```python
from build123d import *

# Parameters (mm, degrees)
F1_DEPTH = 23
F2_DEPTH = 22
F0_W     = 12
F0_H     = 10
F0_R     = 3.5
F3_DEPTH = 16
F4_DEPTH = 18
F5_R     = 0.5
F6_DEPTH = 5


with BuildPart() as f1:
    # F0 (on Top) → F1 (new body)
    with BuildSketch(Plane.XY):
        with BuildLine():
            Line((60, 45), (30, 45))
            Line((30, 45), (30, 41.5))
            Line((30, 41.5), (46, 41.5))
            Line((46, 41.5), (46, 31.5))
            Line((46, 31.5), (46, 22.5))
            Line((46, 22.5), (54.5, 22.5))
            ThreePointArc((54.5, 22.5), (56.1109127035, 26.3890872965), (60, 28))
            Line((60, 28), (60, 31.5))
            Line((60, 31.5), (48, 31.5))
            Line((48, 31.5), (48, 41.5))
            Line((48, 41.5), (60, 41.5))
            Line((60, 41.5), (60, 45))
        make_face()
        with BuildLine():
            Line((54.5, 22.5), (46, 22.5))
            Line((46, 22.5), (46, 13.5))
            Line((46, 13.5), (46, 3.5))
            Line((46, 3.5), (30, 3.5))
            Line((30, 3.5), (30, 0))
            Line((30, 0), (60, 0))
            Line((60, 0), (60, 3.5))
            Line((60, 3.5), (48, 3.5))
            Line((48, 3.5), (48, 13.5))
            Line((48, 13.5), (60, 13.5))
            Line((60, 13.5), (60, 17))
            ThreePointArc((60, 17), (56.1109127035, 18.6109127035), (54.5, 22.5))
        make_face()
        with BuildLine():
            Line((14, 13.5), (14, 22.5))
            Line((14, 22.5), (5.5, 22.5))
            ThreePointArc((5.5, 22.5), (3.8890872965, 18.6109127035), (0, 17))
            Line((0, 17), (0, 13.5))
            Line((0, 13.5), (12, 13.5))
            Line((12, 13.5), (12, 3.5))
            Line((12, 3.5), (0, 3.5))
            Line((0, 3.5), (0, 0))
            Line((0, 0), (30, 0))
            Line((30, 0), (30, 3.5))
            Line((30, 3.5), (14, 3.5))
            Line((14, 3.5), (14, 13.5))
        make_face()
        with BuildLine():
            Line((30, 45), (0, 45))
            Line((0, 45), (0, 41.5))
            Line((0, 41.5), (6, 41.5))
            Line((6, 41.5), (12, 41.5))
            Line((12, 41.5), (12, 31.5))
            Line((12, 31.5), (6, 31.5))
            Line((6, 31.5), (0, 31.5))
            Line((0, 31.5), (0, 28))
            ThreePointArc((0, 28), (3.8890872965, 26.3890872965), (5.5, 22.5))
            Line((5.5, 22.5), (14, 22.5))
            Line((14, 22.5), (14, 31.5))
            Line((14, 31.5), (14, 41.5))
            Line((14, 41.5), (30, 41.5))
            Line((30, 41.5), (30, 45))
        make_face()
    extrude(amount=F1_DEPTH)

    # F0 (on Top) → F2 (join)
    with BuildSketch(Plane.XY):
        Polygon((30, 22.5), (30, 41.5), (14, 41.5), (14, 31.5), (14, 22.5), align=None)
        Polygon((46, 41.5), (30, 41.5), (30, 22.5), (46, 22.5), (46, 31.5), align=None)
        Polygon((46, 22.5), (30, 22.5), (30, 3.5), (46, 3.5), (46, 13.5), align=None)
        Polygon((30, 3.5), (30, 22.5), (14, 22.5), (14, 13.5), (14, 3.5), align=None)
    extrude(amount=F2_DEPTH)

    # F0 (on Top) → F3 (join)
    with BuildSketch(Plane.XY):
        with BuildLine():
            Line((6, 41.5), (0, 41.5))
            Line((0, 41.5), (0, 31.5))
            Line((0, 31.5), (6, 31.5))
            Line((6, 31.5), (6, 33))
            ThreePointArc((6, 33), (2.5, 36.5), (6, 40))
            Line((6, 40), (6, 41.5))
        make_face()
        with BuildLine():
            Line((12, 41.5), (6, 41.5))
            Line((6, 41.5), (6, 40))
            ThreePointArc((6, 40), (8.4748737342, 38.9748737342), (9.5, 36.5))
            ThreePointArc((9.5, 36.5), (8.4748737342, 34.0251262658), (6, 33))
            Line((6, 33), (6, 31.5))
            Line((6, 31.5), (12, 31.5))
            Line((12, 31.5), (12, 41.5))
        make_face()
        with Locations((6, 8.5)):
            Rectangle(F0_W, F0_H)
        with Locations((6, 8.5)):
            Circle(F0_R, mode=Mode.SUBTRACT)
        with Locations((54, 36.5)):
            Rectangle(F0_W, F0_H)
        with Locations((54, 36.5)):
            Circle(F0_R, mode=Mode.SUBTRACT)
        with Locations((54, 8.5)):
            Rectangle(F0_W, F0_H)
        with Locations((54, 8.5)):
            Circle(F0_R, mode=Mode.SUBTRACT)
    extrude(amount=F3_DEPTH)

    # F0 (on Top) → F4 (join)
    with BuildSketch(Plane.XY):
        with BuildLine():
            ThreePointArc((9.5, 36.5), (8.4748737342, 38.9748737342), (6, 40))
            Line((6, 40), (6, 33))
            ThreePointArc((6, 33), (8.4748737342, 34.0251262658), (9.5, 36.5))
        make_face()
        with BuildLine():
            Line((6, 33), (6, 40))
            ThreePointArc((6, 40), (2.5, 36.5), (6, 33))
        make_face()
        with Locations((6, 8.5)):
            Circle(F0_R)
        with Locations((54, 36.5)):
            Circle(F0_R)
        with Locations((54, 8.5)):
            Circle(F0_R)
    extrude(amount=F4_DEPTH)

    # F5
    f5_edges = [f1.edges().sort_by_distance(p)[0] for p in [
        (2.5, 36.5, 18),
        (2.5, 8.5, 18),
        (50.5, 36.5, 18),
        (50.5, 8.5, 18),
    ]]
    fillet(f5_edges, radius=F5_R)

    # F0 (on Top) → F6 (join)
    with BuildSketch(Plane.XY):
        with BuildLine():
            ThreePointArc((5.5, 22.5), (3.8890872965, 26.3890872965), (0, 28))
            Line((0, 28), (0, 22.5))
            Line((0, 22.5), (5.5, 22.5))
        make_face()
        with BuildLine():
            Line((5.5, 22.5), (0, 22.5))
            Line((0, 22.5), (0, 17))
            ThreePointArc((0, 17), (3.8890872965, 18.6109127035), (5.5, 22.5))
        make_face()
        with BuildLine():
            Line((60, 22.5), (60, 28))
            ThreePointArc((60, 28), (56.1109127035, 26.3890872965), (54.5, 22.5))
            Line((54.5, 22.5), (60, 22.5))
        make_face()
        with BuildLine():
            Line((60, 22.5), (54.5, 22.5))
            ThreePointArc((54.5, 22.5), (56.1109127035, 18.6109127035), (60, 17))
            Line((60, 17), (60, 22.5))
        make_face()
    extrude(amount=F6_DEPTH)


solid = f1.part
```
Read the model definition and answer for the solid it produces. Units are mm, in the model's axes. A direction names the side the tool comes from. Give positions to 0.01 mm unless a question says otherwise; leave off trailing zeros. Order: outer loops, then holes, each group sorted by start corner. A loop starts at its lowest first (then second) coordinate and runs counter-clockwise, first axis right, second up. Notation, with made-up numbers: (33, 10.25) -> (72, 10.25) arc R26 cw to (72, 39.25) -> close; hole circle Ø2 at (69, 75.25). An arc over 180 degrees is marked (long way). Write item = value, one per line.
1. A cutting plane is placed at B-B, the plane z = 18.75. Write down the section's boundary in (x, y).
Numbers:
outline = (0, 0) -> (60, 0) -> (60, 3.5) -> (48, 3.5) -> (48, 13.5) -> (60, 13.5) -> (60, 17) arc R5.5 cw to (60, 28) -> (60, 31.5) -> (48, 31.5) -> (48, 41.5) -> (60, 41.5) -> (60, 45) -> (0, 45) -> (0, 41.5) -> (12, 41.5) -> (12, 31.5) -> (0, 31.5) -> (0, 28) arc R5.5 cw to (0, 17) -> (0, 13.5) -> (12, 13.5) -> (12, 3.5) -> (0, 3.5) -> close
2. A cutting plane is placed at D-D, the plane y = 18. Write down the section's boundary in (x, z).
Numbers:
outline = (0, 0) -> (60, 0) -> (60, 5) -> (56.84, 5) -> (56.84, 23) -> (46, 23) -> (46, 22) -> (14, 22) -> (14, 23) -> (3.16, 23) -> (3.16, 5) -> (0, 5) -> close
3. Given pin 1 (2 mm diameter, centred on y = 37, z = 18.5, fed in from -X); pin 2 (3 mm diameter, centred on x = 55.5, y = 8.5, fed in from +Z); pin 3 (0.5 mm diameter, centred on y = 18.5, z = 22.5, fed in from +X), each flat-ended and moving along its own axis, determine where each tip first touches the part or whether it passes through.
Numbers:
pin_1 = 2.51
pin_2 = 18
pin_3 = 56.51
4. For faces 5 (the face through (3, 39, 16)), 6 (the face through (12, 21, 23)), 7 (the face through (2, 23, 5)), 8 (the face through (54, 9, 18)), determine the directions among +Z, -Z, +X, -X, +Y, -Y from which every point of the face is accessible in a straight line to the end or side of a thin tool.
Numbers:
face_5 = +Z
face_6 = +Z, +X, -X, +Y, -Y
face_7 = +Z, -X
face_8 = +Z, +X
5. A cutting plane is placed at C-C, the plane y = 8.5. Write down the section's boundary in (x, z), and give its area (3 significant figures).
Numbers:
outline = (0, 0) -> (60, 0) -> (60, 16) -> (57.5, 16) -> (57.5, 17.5) arc R0.5 ccw to (57, 18) -> (51, 18) arc R0.5 ccw to (50.5, 17.5) -> (50.5, 16) -> (48, 16) -> (48, 23) -> (46, 23) -> (46, 22) -> (14, 22) -> (14, 23) -> (12, 23) -> (12, 16) -> (9.5, 16) -> (9.5, 17.5) arc R0.5 ccw to (9, 18) -> (3, 18) arc R0.5 ccw to (2.5, 17.5) -> (2.5, 16) -> (0, 16) -> close
area = 1,210 mm²
6. A cutting plane is placed at A-A, the plane x = 30. Write down the section's boundary in (y, z), and give its area (3 significant figures).
Numbers:
outline = (0, 0) -> (45, 0) -> (45, 23) -> (41.5, 23) -> (41.5, 22) -> (3.5, 22) -> (3.5, 23) -> (0, 23) -> close
area = 997 mm²
7. The mould has two halves that part along Y. Classify faces 1 (the face through (60, 22, 4)), 2 (the face through (6, 37, 18)), 3 (the face through (30, 45, 11)), 4 (the face through (7.615, 5.395, 16.74)): +Y half, -Y half, draft (parallel to the pull), parting line (faces both ways), or undercut.
Numbers:
face_1 = draft
face_2 = undercut
face_3 = +Y half
face_4 = undercut
8. Straight lines are drawn through the part: line 1 along X through (y, z) = (34.5, 17.75); line 2 along Z through (x, y) = (7, 7); line 3 along Z through (x, y) = (28.5, 15). For each, find the intervals that lie inside material, in ascending order.
Numbers:
line_1 = 3.21 to 8.79, 12 to 48, 51.21 to 56.79
line_2 = 0 to 18
line_3 = 0 to 22
